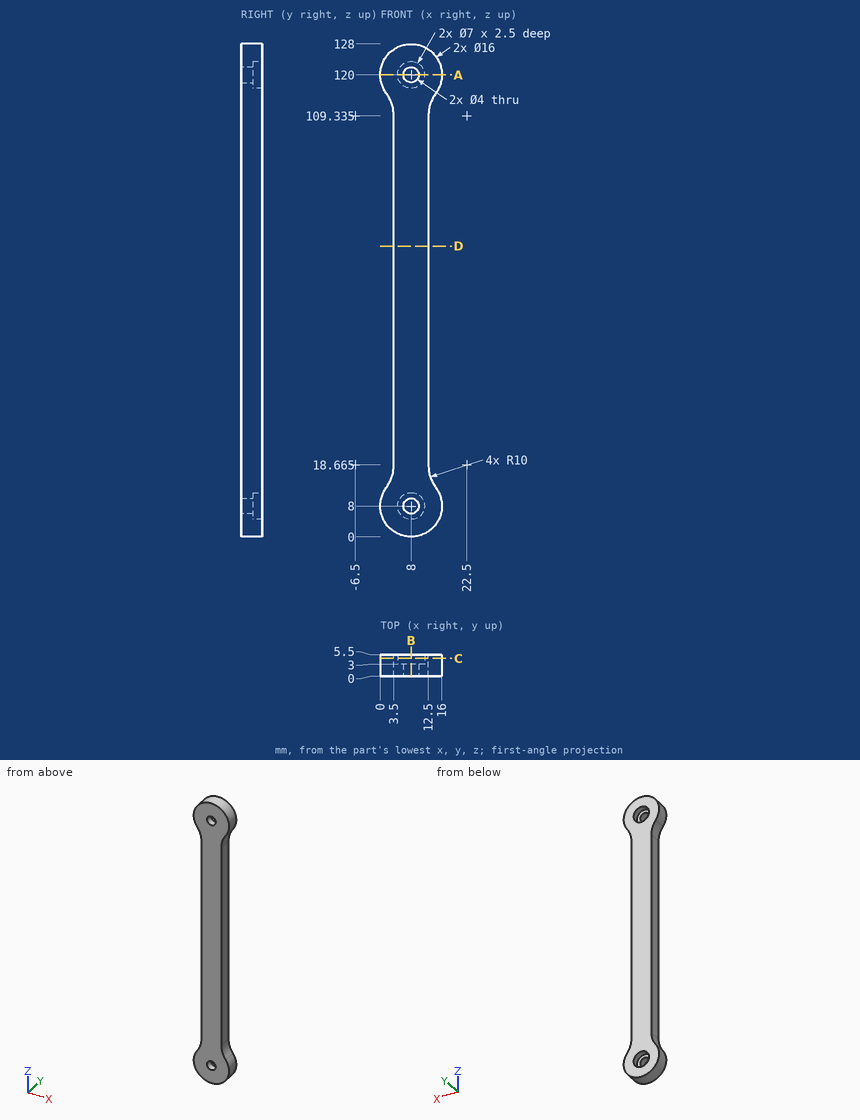
Answer from the drawing. Dimensions are ordinates in mm from the lowest x, y and z of the part. Round coordinates to 2 decimals unless told otherwise and drop trailing zeros. Write each loop counter-clockwise with the first axis right and the second up, starting at its lowest first coordinate (ties: lowest second). Pieces come first, ordered by that corner, then holes. Notation, with made-up numbers: (30, 13) - (36, 13) arc R18 cw to (36, 25) - close; hole circle Ø8 at (34, 7). An arc over 180 degrees is marked (long way). Use a Markdown table: item, result.
(1) Each of these flat-tipped pins is pushed along its axis until it touches: pin 1 Ø1.6 at (y, z) = (3.5, 66) entering from -X; pin 2 Ø3 at (y, z) = (4, 41.5) entering from +X; pin 3 Ø2.5 at (x, z) = (8, 8) entering from +Y. Where does it stop, or does it pass through?
Reported:
| item | result |
|---|---|
| pin 1 | x = 3.5 |
| pin 2 | x = 12.5 |
| pin 3 | through |
(2) Straight lines are drawn through the part: line 1 along Z through (x, y) = (8, 0.75); line 2 along Z through (x, y) = (8, 4.8); line 3 along X through (y, z) = (1.2, 120). For each, find the intervals that lie inside material, in ascending order. Write a range as [from, to].
Reported:
| item | result |
|---|---|
| line 1 | [0, 6], [10, 118], [122, 128] |
| line 2 | [0, 4.5], [11.5, 116.5], [123.5, 128] |
| line 3 | [0, 6], [10, 16] |
(3) The part is cut by section D-D (z = 75.5). Write down the section's boundary in (x, y), then the cut area to 3 significant figures.
Reported:
| item | result |
|---|---|
| outline | (3.5, 0) - (12.5, 0) - (12.5, 5.5) - (3.5, 5.5) - close |
| area | 49.5 mm2 |
(4) The part is cut by section C-C (y = 4.6). Write down the section's boundary in (x, z) (1 decimal), then the cut area to 3 significant figures.
Reported:
| item | result |
|---|---|
| outline | (1.6, 12.7) arc R8 ccw (long way) to (14.4, 12.7) arc R10 cw to (12.5, 18.7) - (12.5, 109.3) arc R10 cw to (14.4, 115.3) arc R8 ccw (long way) to (1.6, 115.3) arc R10 cw to (3.5, 109.3) - (3.5, 18.7) arc R10 cw to start; hole circle Ø7 at (8, 8); hole circle Ø7 at (8, 120) |
| area | 1,200 mm2 |
(5) The part is cut by section A-A (z = 120). Write down the section's boundary in (x, y), then the cut area to 3 significant figures.
Reported:
| item | result |
|---|---|
| outline | (0, 0) - (6, 0) - (6, 3) - (4.5, 3) - (4.5, 5.5) - (0, 5.5) - close; (10, 0) - (16, 0) - (16, 5.5) - (11.5, 5.5) - (11.5, 3) - (10, 3) - close |
| area | 58.5 mm2 |
(6) The part is cut by section B-B (x = 8). Write down the section's boundary in (y, z).
Reported:
| item | result |
|---|---|
| outline | (0, 0) - (5.5, 0) - (5.5, 4.5) - (3, 4.5) - (3, 6) - (0, 6) - close; (0, 10) - (3, 10) - (3, 11.5) - (5.5, 11.5) - (5.5, 116.5) - (3, 116.5) - (3, 118) - (0, 118) - close; (0, 122) - (3, 122) - (3, 123.5) - (5.5, 123.5) - (5.5, 128) - (0, 128) - close |
